Design review of the part built by this model. Coordinates are the model's own, in mm. Face numbers are marked on the shaded views. A direction names the side the tool comes from. Round coordinates to 2 decimals unless told otherwise and drop trailing zeros. Loops run counter-clockwise (first coordinate to the right, second up) from the corner with the lowest first, then second, coordinate; pieces in that order, holes last. Notation, with made-up numbers: (78.25, 8.5) - (107.25, 8.5) arc R8 ccw to (107.25, 16.5) - close; hole circle Ø5 at (-9, -8). An arc over 180 degrees is marked (long way). Return JSON: item names as keys, results as strings. Group by question number.
from build123d import *

# Parameters (mm, degrees)
SKETCH2_W           = 30
SKETCH2_H           = 20
BOSS_EXTRUDE1_DEPTH = 50
SKETCH3_R           = 14.125
CUT_EXTRUDE1_DEPTH  = 16
SKETCH4_R           = 3.25
CUT_EXTRUDE2_DEPTH  = 16


with BuildPart() as part:
    # Sketch2 → Boss-Extrude1 (new body)
    with BuildSketch(Plane.XY):
        with Locations((15, 10)):
            Rectangle(SKETCH2_W, SKETCH2_H)
    extrude(amount=BOSS_EXTRUDE1_DEPTH)

    # Sketch3 → Cut-Extrude1 (cut)
    with BuildSketch(Plane(origin=(0, 20, 0), x_dir=(1, 0, 0), z_dir=(0, 1, 0))):
        with Locations(Location((15, -25, 0), (0, 0, 270))):
            Circle(SKETCH3_R)
    extrude(amount=-CUT_EXTRUDE1_DEPTH, mode=Mode.SUBTRACT)

    # Sketch4 → Cut-Extrude2 (cut)
    with BuildSketch(Plane(origin=(0, 4, 0), x_dir=(1, 0, 0), z_dir=(0, 1, 0))):
        with Locations(Location((15, -25, 0), (0, 0, 270))):
            Circle(SKETCH4_R)
    extrude(amount=-CUT_EXTRUDE2_DEPTH, mode=Mode.SUBTRACT)


solid = part.part
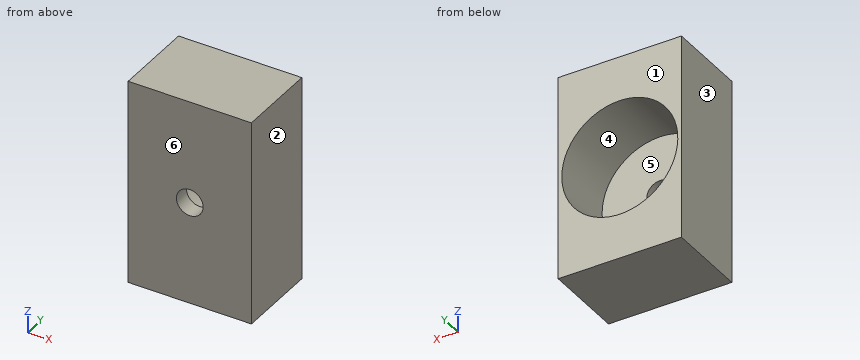
Q1. Tool access review of the marked faces 5 and 6: name each direction out of +Z, -Z, +X, -X, +Y, -Y from which nothing blocks a thin tool from reaching the whole face with its end or side.
Q2. Draft analysis for pull direction X (two halves, no side actions). For the marked faces 1, 2, 3 and 4, state which applies: pulls with the +X half, pulls with the -X half, needs draft (parallel to the pull), parting line crosses it, or undercut.
Q3. Insertion check: pin 1 Ø1.5 at (x, z) = (13, 33.5) entering from +Y. The pin has a flat end and moves straight along its axis. Give the tip position at first contact, or say it passes through.
Q4. Add section A-A, the plane z = 25. State the section outline as (x, y) points (3 decimals).
Q5. Add section B-B, the plane x = 15. State the section outline as (y, z) points (3 decimals), plus the area to 3 significant figures.
Q6. Add section D-D, the plane z = 32. State the section outline as (x, y) points, plus the area to 3 significant figures.
Q7. For line 1 (X direction, y = 12.25, z = 25) (3 decimals); line 2 (X direction, y = 1.9, z = 25); line 3 (Y direction, x = 28, z = 28), list the stretches that pass through material, from the lowest coordinate up.
Q8. Add section C-C, the plane y = 1.5. State the section outline as (x, z) points.
Evaluation:
{
 "1": {"face 5": "+Y", "face 6": "+Z, -Z, +X, -X, -Y"},
 "2": {"face 1": "needs draft", "face 2": "pulls with the +X half", "face 3": "pulls with the -X half", "face 4": "undercut"},
 "3": {"pin 1": "y = 4"},
 "4": {"outline": "(0, 0) - (11.75, 0) - (11.75, 4) - (0.875, 4) - (0.875, 20) - (0, 20) - close; (18.25, 0) - (30, 0) - (30, 20) - (29.125, 20) - (29.125, 4) - (18.25, 4) - close"},
 "5": {"outline": "(0, 0) - (20, 0) - (20, 10.875) - (4, 10.875) - (4, 21.75) - (0, 21.75) - close; (0, 28.25) - (4, 28.25) - (4, 39.125) - (20, 39.125) - (20, 50) - (0, 50) - close", "area": "522 mm²"},
 "6": {"outline": "(0, 0) - (30, 0) - (30, 20) - (27.27, 20) - (27.27, 4) - (2.73, 4) - (2.73, 20) - (0, 20) - close", "area": "207 mm²"},
 "7": {"line 1": "0 to 0.875, 29.125 to 30", "line 2": "0 to 11.75, 18.25 to 30", "line 3": "0 to 4"},
 "8": {"outline": "(0, 0) - (30, 0) - (30, 50) - (0, 50) - close; hole circle Ø6.5 at (15, 25)"}
}
